```python
from build123d import *

# Parameters (mm, degrees)
BOSS_EXTRUDE1_DEPTH = 10
FILLET1_R           = 7
BOSS_EXTRUDE2_DEPTH = 2.5
SKETCH8_W           = 6
SKETCH8_H           = 16
CUT_EXTRUDE1_DEPTH  = 6
SKETCH9_R           = 12
BOSS_EXTRUDE3_DEPTH = 2.5
SKETCH10_R          = 10.5
CUT_EXTRUDE2_DEPTH  = 6


with BuildPart() as part:
    # Sketch1 → Boss-Extrude1 (new body)
    with BuildSketch(Plane.XY):
        with BuildLine():
            Line((0, 0), (67.8, 0))
            ThreePointArc((67.8, 0), (72.369764115, -34.141185106), (70.341123561, -68.527052581))
            ThreePointArc((70.341123561, -68.527052581), (51.546832931, -107.857068487), (14.233546266, -130.391356799))
            ThreePointArc((14.233546266, -130.391356799), (7.138727746, -132.120022188), (0, -133.657325027))
            Line((0, -133.657325027), (0, 0))
        make_face()
    extrude(amount=BOSS_EXTRUDE1_DEPTH)

    # Fillet1
    fillet1_edges = [part.edges().sort_by_distance(p)[0] for p in [
        (72.369764115, -34.141185106, 0),
        (51.546832931, -107.857068487, 0),
        (7.138727746, -132.120022188, 0),
    ]]
    fillet(fillet1_edges, radius=FILLET1_R)

    # Sketch7 → Boss-Extrude2 (add)
    with BuildSketch(Plane.XY.offset(10)):
        with BuildLine():
            Line((11, -11), (11, -119.864879644))
            ThreePointArc((11, -119.864879644), (11.243089625, -119.802551163), (11.486119117, -119.739988621))
            ThreePointArc((11.486119117, -119.739988621), (32.734504551, -109.903861987), (49.119007756, -93.176897964))
            ThreePointArc((49.119007756, -93.176897964), (38.323820757, -73.187087964), (59.682991081, -65.446648104))
            ThreePointArc((59.682991081, -65.446648104), (61.472976924, -38.189093901), (58.840205899, -11))
            Line((58.840205899, -11), (11, -11))
        make_face()
    extrude(amount=BOSS_EXTRUDE2_DEPTH)

    # Sketch8 → Cut-Extrude1 (cut)
    with BuildSketch(Plane.XY.offset(10)):
        with Locations((5, -115.657325027)):
            Rectangle(SKETCH8_W, SKETCH8_H)
    extrude(amount=-CUT_EXTRUDE1_DEPTH, mode=Mode.SUBTRACT)

    # Sketch9 → Boss-Extrude3 (add)
    with BuildSketch(Plane.XY.offset(10)):
        with Locations((52.341123561, -78.527052581)):
            Circle(SKETCH9_R)
    extrude(amount=BOSS_EXTRUDE3_DEPTH)

    # Sketch10 → Cut-Extrude2 (cut)
    with BuildSketch(Plane.XY.offset(12.5)):
        with Locations((52.341123561, -78.527052581)):
            Circle(SKETCH10_R)
    extrude(amount=-CUT_EXTRUDE2_DEPTH, mode=Mode.SUBTRACT)


solid = part.part
```
Could you check a few things on this model? Use its own coordinates, in mm. A direction names the side the tool comes from. Round coordinates to 2 decimals unless told otherwise and drop trailing zeros. Write each loop counter-clockwise with the first axis right and the second up, starting at its lowest first coordinate (ties: lowest second). Pieces come first, ordered by that corner, then holes.
(1) Suppose I cut it at A-A on z = 11.25. Write out the boundary of the cut face in (x, y), and give its area (3 significant figures).
Findings below:
outline: (11, -119.86) arc R260.6 ccw to (11.49, -119.74) arc R65 ccw to (49.12, -93.18) arc R15 cw (long way) to (59.68, -65.45) arc R168.69 ccw to (58.84, -11) - (11, -11) - close; circle Ø24 at (52.34, -78.53); hole circle Ø21 at (52.34, -78.53)
area: 4,240 mm2
(2) For pin 1 (1.8 mm diameter, centred on x = 4.5, y = -113, fed in from +Z); pin 2 (1.8 mm diameter, centred on x = 4, z = 8.5, fed in from -Y); pin 3 (6.5 mm diameter, centred on x = 56.5, y = -78, fed in from +Z); pin 4 (12 mm diameter, centred on x = 20, y = -40, fed in from -Z), each with a flat end and sliding along its axis, tell me the tip position at first contact or that it passes through.
Findings below:
pin 1: stops at z = 4
pin 2: stops at y = -133.01
pin 3: stops at z = 6.5
pin 4: stops at z = 0
(3) If I drill on probe 1 along Y at (x, z) = (45.5, 11); probe 2 along X at (y, z) = (-78, 7); probe 3 along Z at (x, y) = (48, -75.5), over which ranges is the centre line in solid material (lowest first)?
Findings below:
probe 1: y = -98.03 to -91.88, -88.39 to -86.49, -70.56 to -68.67, -65.18 to -11
probe 2: x = 0 to 41.85, 62.83 to 68.23
probe 3: z = 0 to 6.5
(4) Which directions (+Z, -Z, +X, -X, +Y, -Y) give clear straight access to the entire face, cutting with the end or side of a thin tool? Please do faces 1 (the face through (32.465, -110.093, 11.232)), 2 (the face through (11, -65, 11)), 3 (the face through (5, -123.657, 7)).
Findings below:
face 1: +Z, +X, -Y
face 2: +Z, -X, +Y, -Y
face 3: +Z
